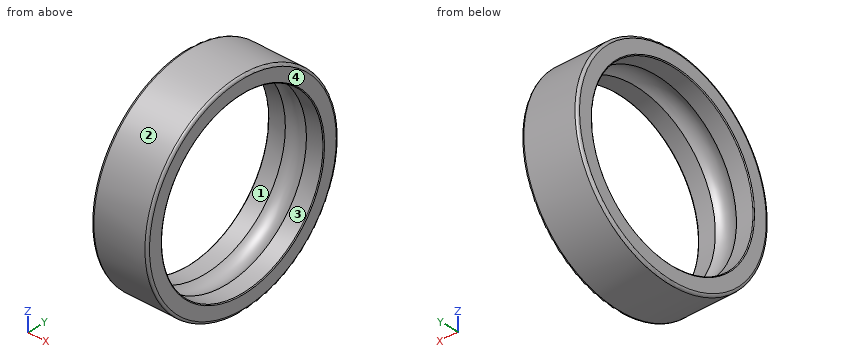
Autodesk Inventor part; units mm, degrees
ref_plane "YZ Plane" through (0, 0, 0) normal (1, 0, 0) x (0, 1, 0)
ref_plane "XZ Plane" through (0, 0, 0) normal (0, 1, 0) x (-1, 0, 0)
ref_plane "XY Plane" through (0, 0, 0) normal (0, 0, 1) x (1, 0, 0)
sketch "Sketch_1" plane through (0, 0, 0) normal (0, 0, 1) x (1, 0, 0)
  line L0 (50, 0) -> (-50, 0)
  line L1 (0, 6.35) -> (0, 5.55)
  arc A0 (0, 5.55) -> (0.05, 5.5) centre (0.05, 5.55) ccw
  line L2 (0.05, 5.5) -> (1.0886, 5.5)
  arc A1 (2.4114, 5.5) -> (1.0886, 5.5) centre (1.75, 4.75) ccw
  line L3 (2.4114, 5.5) -> (3.45, 5.5)
  arc A2 (3.45, 5.5) -> (3.5, 5.55) centre (3.45, 5.55) ccw
  line L4 (3.5, 5.55) -> (3.5, 6.35)
  arc A3 (3.5, 6.35) -> (3.35, 6.5) centre (3.35, 6.35) ccw
  line L5 (3.35, 6.5) -> (0.15, 6.5)
  arc A4 (0.15, 6.5) -> (0, 6.35) centre (0.15, 6.35) ccw
revolve "Revolution1" add sketch "Sketch_1" angle 360 about axis through (50, 0, 0) along (1, 0, 0)
properties part number "SKF_618/6_PART2"
Verification items for the finished model (mm, model axes). Face numbers are marked on the shaded views. Coordinates: 2 decimals unless noted, no trailing zeros. Order: outer loops, then holes, each group sorted by start corner. A loop starts at its lowest first (then second) coordinate and runs counter-clockwise, first axis right, second up. Notation, with made-up numbers: M 61,52.5 L 99,52.5 A5 ccw 99,58.5 Z; hole C 61.25,7 d7. An arc over 180 degrees is marked long. One line per item, written item: value. Start each with the question number.
Item 1: Sectioned sample at D-D (x = 1.5). Enter the section's corners in (y, z), then the cut area to 3 significant figures.
Item 2: Mould release check, pull along Y, two halves, no side actions. Record for the marked faces 1, 2, 3 and 4: released by +Y, released by -Y, zero draft, split by the parting line, or undercut.
Item 3: Gauge pin test, flat ends, axial feed: pin 1 (1 mm diameter, centred on x = 0.5, z = 4, fed in from +Y); pin 2 (1 mm diameter, centred on x = 1.5, y = -4, fed in from -Z); pin 3 (2 mm diameter, centred on x = 2.5, y = -1.5, fed in from -Z); pin 4 (5 mm diameter, centred on y = -4, z = -1.5, fed in from +X). Record the tip position at first contact, or that the pin passes through.
Item 4: Sectioned sample at A-A (z = 0). Enter the section's corners in (x, y).
Item 5: Sectioned sample at C-C (x = 2.75). Enter the section's corners in (y, z).
Item 6: Scan lines: probe 1 along Z at (x, y) = (2.7, 0); probe 2 along Z at (x, y) = (2.05, -4.25); probe 3 along Y at (x, z) = (2.55, 3). Record each from-to range of solid material in increasing order.
Conclusion:
1. outline: C 0,0 d13; hole C 0,0 d11.44
1. area: 30.0 mm^2
2. face 1: undercut
2. face 2: split by the parting line
2. face 3: undercut
2. face 4: zero draft
3. pin 1: stops at y = 5.48
3. pin 2: stops at z = -5.48
3. pin 3: stops at z = -6.48
3. pin 4: stops at x = 3.5
4. outline: M 0,-6.35 A0.15 ccw 0.15,-6.5 L 3.35,-6.5 A0.15 ccw 3.5,-6.35 L 3.5,-5.55 A0.05 ccw 3.45,-5.5 L 2.41,-5.5 A1 cw 1.09,-5.5 L 0.05,-5.5 A0.05 ccw 0,-5.55 Z; M 0,5.55 A0.05 ccw 0.05,5.5 L 1.09,5.5 A1 cw 2.41,5.5 L 3.45,5.5 A0.05 ccw 3.5,5.55 L 3.5,6.35 A0.15 ccw 3.35,6.5 L 0.15,6.5 A0.15 ccw 0,6.35 Z
5. outline: C 0,0 d13; hole C 0,0 d11
6. probe 1: z = -6.5 to -5.5, 5.5 to 6.5
6. probe 2: z = -4.92 to -3.8, 3.8 to 4.92
6. probe 3: y = -5.77 to -4.61, 4.61 to 5.77
